from build123d import *

# Parameters (mm, degrees)
F0_W     = 8.128
F0_H     = 29.972
F0_R     = 1.41732
F1_DEPTH = 1.5875
F2_W     = 3.175
F2_H     = 3.175
F3_DEPTH = 1.5875


with BuildPart() as f1:
    # F0 (on Front) → F1 (new body)
    with BuildSketch(Plane.XZ):
        Rectangle(F0_W, F0_H)
        Circle(F0_R, mode=Mode.SUBTRACT)
    extrude(amount=F1_DEPTH)

    # F2 (on face) → F3 (join)
    with BuildSketch(Plane(origin=(0, 0, 0), x_dir=(-1, 0, 0), z_dir=(0, 1, 0))):
        with Locations((0, 13.3985)):
            Rectangle(F2_W, F2_H)
    extrude(amount=F3_DEPTH)


solid = f1.part
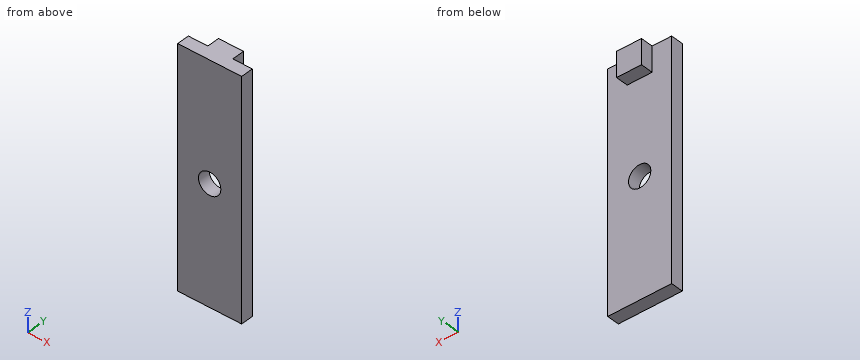
Work out the finished part from the listing and answer in its coordinate system (mm). Round coordinates to 2 decimals unless told otherwise and drop trailing zeros. Write each loop counter-clockwise with the first axis right and the second up, starting at its lowest first coordinate (ties: lowest second). Pieces come first, ordered by that corner, then holes. Notation, with made-up numbers: (5, 27.5) - (58, 27.5) arc R20 ccw to (58, 42.5) - close; hole circle Ø1 at (3, -20). An arc over 180 degrees is marked (long way). Answer in a Markdown table with one row per item. Add a question column.
1. A cutting plane is placed at C-C, the plane y = -0.45. Determine the outline of the cut face in (x, z).
2. Find the intervals of material crossed by line 1 along Z through (x, y) = (0, -0.25); line 2 along Z through (x, y) = (-1.25, -0.2); line 3 along X through (y, z) = (0.05, 13.5), in increasing order. Write a range as from..to.
3. A cutting plane is placed at D-D, the plane x = -3.25. Determine the outline of the cut face in (y, z).
4. A cutting plane is placed at A-A, the plane x = 0. Determine the outline of the cut face in (y, z), and give its area (3 significant figures).
5. Given pin 1 (1.3 mm diameter, centred on y = 0.5, z = 14, fed in from -X); pin 2 (1.7 mm diameter, centred on x = 0, z = 0, fed in from -Y); pin 3 (4 mm diameter, centred on x = -1, z = 8, fed in from +Y); pin 4 (0.8 mm diameter, centred on x = -0.5, y = 0.5, fed in from -Z), each flat-ended and moving along its own axis, determine where each tip first touches the part or whether it passes through.
6. A cutting plane is placed at B-B, the plane z = 0. Determine the outline of the cut face in (x, y), and give its area (3 significant figures).
Worked out:
| question | item | result |
|---|---|---|
| 1 | outline | (-4.06, -14.99) - (4.06, -14.99) - (4.06, 14.99) - (-4.06, 14.99) - close; hole circle Ø2.83 at (0, 0) |
| 2 | line 1 | -14.99..-1.42, 1.42..14.99 |
| 2 | line 2 | -14.99..-0.67, 0.67..14.99 |
| 2 | line 3 | -1.59..1.59 |
| 3 | outline | (-1.59, -14.99) - (0, -14.99) - (0, 14.99) - (-1.59, 14.99) - close |
| 4 | outline | (-1.59, -14.99) - (0, -14.99) - (0, -1.42) - (-1.59, -1.42) - close; (-1.59, 1.42) - (0, 1.42) - (0, 11.81) - (1.59, 11.81) - (1.59, 14.99) - (-1.59, 14.99) - close |
| 4 | area | 48.1 mm^2 |
| 5 | pin 1 | x = -4.06 |
| 5 | pin 2 | through |
| 5 | pin 3 | y = 0 |
| 5 | pin 4 | z = 11.81 |
| 6 | outline | (-4.06, -1.59) - (-1.42, -1.59) - (-1.42, 0) - (-4.06, 0) - close; (1.42, -1.59) - (4.06, -1.59) - (4.06, 0) - (1.42, 0) - close |
| 6 | area | 8.40 mm^2 |
